Source: CAD feature listing. Evaluate the final solid. Frame: model axes, mm. Face numbers are marked on the shaded views. Round coordinates to 2 decimals unless told otherwise and drop trailing zeros. Order: outer loops, then holes, each group sorted by start corner. A loop starts at its lowest first (then second) coordinate and runs counter-clockwise, first axis right, second up. Notation, with made-up numbers: (3.5, 74.25) -> (58.5, 74.25) arc R16 ccw to (58.5, 102.25) -> close; hole circle Ø11 at (63, 74). An arc over 180 degrees is marked (long way). Answer as CSV lines item,"result".
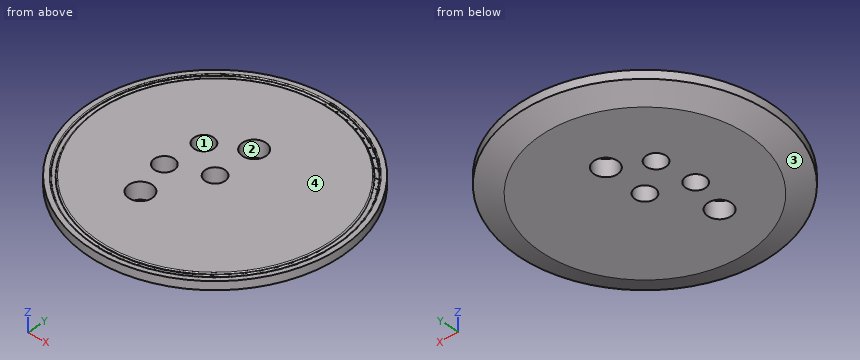
from build123d import *

# Parameters (mm, degrees)
SKETCH2_R          = 6.5
SKETCH2_R_2        = 7.75
CUT_EXTRUDE1_DEPTH = 119.521470637


with BuildPart() as part:
    # Sketch1 → Revolve1 (revolve)
    with BuildSketch(Plane(origin=(0, 0, 0), x_dir=(0, 0, -1), z_dir=(1, 0, 0)), mode=Mode.PRIVATE) as revolve1_sk:
        with BuildLine():
            Line((0, 0), (0, 76.444627725))
            ThreePointArc((0, 76.444627725), (0.130798304, 76.879222907), (0.479738309, 77.169433247))
            Line((0.479738309, 77.169433247), (0.872854821, 77.336301306))
            ThreePointArc((0.872854821, 77.336301306), (1.6002, 78.4352), (0.872854821, 79.534098694))
            Line((0.872854821, 79.534098694), (0.479738309, 79.700966753))
            ThreePointArc((0.479738309, 79.700966753), (0.130798304, 79.991177093), (0, 80.425772275))
            Line((0, 80.425772275), (0, 83.439))
            Line((0, 83.439), (5.588, 83.439))
            Line((5.588, 83.439), (11.0998, 68.295453959))
            Line((11.0998, 68.295453959), (11.0998, 0))
            Line((11.0998, 0), (0, 0))
        make_face()
    revolve(revolve1_sk.sketch.rotate(Axis((0, 0, 0), (0, 0, -1)), 90), axis=Axis((0, 0, 0), (0, 0, -1)))

    # Sketch2 → Cut-Extrude1 (cut, through all)
    with BuildSketch(Plane(origin=(0, 0, -11.0998), x_dir=(-1, 0, 0), z_dir=(0, 0, -1))):
        Circle(SKETCH2_R)
        with Locations((0, 27.9765569)):
            Circle(SKETCH2_R_2)
        with Locations((24.098999837, -10.15759269)):
            Circle(SKETCH2_R)
        with Locations((21.259374059, 15.100131331)):
            Circle(SKETCH2_R)
        with Locations((18.120840305, -33.771322839)):
            Circle(SKETCH2_R_2)
    extrude(amount=-CUT_EXTRUDE1_DEPTH, mode=Mode.SUBTRACT)


solid = part.part
1. Mould query, pull axis Y, two halves, no side actions, for the marked faces 1, 2, 3 and 4. Classes: released by +Y, released by -Y, zero draft, split by the parting line, or undercut.
Results below:
face 1,"undercut"
face 2,"undercut"
face 3,"split by the parting line"
face 4,"zero draft"
2. Section query A-A on x = 0. Return loops of the section in (y, z).
Results below:
outline,"(-83.44, -5.59) -> (-68.3, -11.1) -> (-6.5, -11.1) -> (-6.5, 0) -> (-76.44, 0) arc R0.79 ccw to (-77.17, -0.48) -> (-77.34, -0.87) arc R1.19 cw to (-79.53, -0.87) -> (-79.7, -0.48) arc R0.79 ccw to (-80.43, 0) -> (-83.44, 0) -> close; (6.5, -11.1) -> (20.23, -11.1) -> (20.23, 0) -> (6.5, 0) -> close; (35.73, -11.1) -> (68.3, -11.1) -> (83.44, -5.59) -> (83.44, 0) -> (80.43, 0) arc R0.79 ccw to (79.7, -0.48) -> (79.53, -0.87) arc R1.19 cw to (77.34, -0.87) -> (77.17, -0.48) arc R0.79 ccw to (76.44, 0) -> (35.73, 0) -> close"
3. Section query C-C on z = -3.5. Return loops of the section in (x, y).
Results below:
outline,"circle Ø166.88 at (0, 0); hole circle Ø13 at (-24.1, -10.16); hole circle Ø13 at (-21.26, 15.1); hole circle Ø15.5 at (-18.12, -33.77); hole circle Ø15.5 at (0, 27.98); hole circle Ø13 at (0, 0)"
4. Section query B-B on y = 0. Return loops of the section in (x, z), and give its area (3 significant figures).
Results below:
outline,"(-83.44, -5.59) -> (-68.3, -11.1) -> (-6.5, -11.1) -> (-6.5, 0) -> (-76.44, 0) arc R0.79 ccw to (-77.17, -0.48) -> (-77.34, -0.87) arc R1.19 cw to (-79.53, -0.87) -> (-79.7, -0.48) arc R0.79 ccw to (-80.43, 0) -> (-83.44, 0) -> close; (6.5, -11.1) -> (68.3, -11.1) -> (83.44, -5.59) -> (83.44, 0) -> (80.43, 0) arc R0.79 ccw to (79.7, -0.48) -> (79.53, -0.87) arc R1.19 cw to (77.34, -0.87) -> (77.17, -0.48) arc R0.79 ccw to (76.44, 0) -> (6.5, 0) -> close"
area,"1,620 mm2"
5. Pin query (flat end, axial travel): pin 1 (4 mm diameter, centred on x = 5.5, z = -4.5, fed in from +Y); pin 2 (5 mm diameter, centred on x = 37, z = -1, fed in from -Y); pin 3 (12 mm diameter, centred on x = 64.5, y = -38.5, fed in from -Z). Return the tip coordinate at first contact, or that it passes through.
Results below:
pin 1,"y = 83.37"
pin 2,"y = -75.97"
pin 3,"z = -10.8"
6. Line query: L1, parallel to Y at x = -26.5, z = -3.25; L2, parallel to X at y = 51, z = -0.25; L3, parallel to X at y = -20.5, z = -2.5. Output: solid intervals per line, ascending. Write a range as [from, to].
Results below:
L1,"[-79.12, -16.2], [-4.12, 11.25], [18.95, 79.12]"
L2,"[-66.04, -61.44], [-57.72, 57.72], [61.44, 66.04]"
L3,"[-80.88, 80.88]"
